Design review of the part built by this model. Coordinates are the model's own, in mm. Face numbers are marked on the shaded views. A direction names the side the tool comes from. Coordinates: 2 decimals unless noted, no trailing zeros. Write each loop counter-clockwise with the first axis right and the second up, starting at its lowest first coordinate (ties: lowest second). Pieces come first, ordered by that corner, then holes.
Solid Edge part; units mm, degrees
sketch "Sketch1" plane through (0, 0, 0) normal (0, -1, 0) x (1, 0, 0)
  line L0 (0, 12) -> (6, 12)
  line L1 (6, 12) -> (6, 10)
  line L2 (6, 10) -> (4, 10)
  line L3 (4, 10) -> (4, 0)
  line L4 (4, 0) -> (0, 0)
  line L5 (0, 0) -> (0, 12)
revolve "RevolvedProtrusion1" add sketch "Sketch1" angle 360 about axis through (0, 0, 0) along (0, 0, 1)
chamfer "Chamfer1" distance 1.5 angle 45 1 edges at (-6, 0, 12)
chamfer "Chaflán_2" distance 0.5 angle 45 1 edges at (-4, 0, 0)
sketch "Sketch2" plane through (0, 0, 10) normal (0, 0, -1) x (1, 0, 0)
  line L0 (1.5, 7) -> (-1.5, 7)
  line L1 (-1.5, 7) -> (-1.5, 5)
  line L2 (-1.5, 5) -> (1.5, 5)
  line L3 (1.5, 5) -> (1.5, 7)
extrude "VaciadoExtruido_1" cut sketch "Sketch2" against normal blind 0.5
pattern_circular "Pattern1" count 3 over 360 about axis through (0, 0, 10) along (0, 0, -1) of "VaciadoExtruido_1"
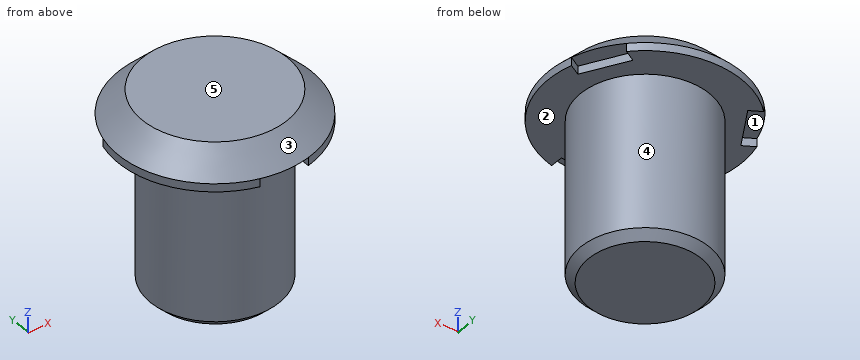
(1) Consider section B-B (y = 0). Give the boundary of the cut face in (x, z).
(2) Wall thickness on line 1 (Y direction, x = 0, z = 3.5); line 2 (Z direction, x = -0.5, y = -4); line 3 (Z direction, x = -4.25, y = -4): over which ranges is each line inside the solid? List them lowest first.
(3) For the marked faces 4 and 5, list the 3-axis set-ups (+Z, -Z, +X, -X, +Y, -Y) from which the entire face can be reached by the end or side of a thin tool; tool diameter is ignored.
(4) Mouldability with a two-part tool opening along Y and no side actions: class the marked faces 1, 2 and 3 as +Y half, -Y half, draft (parallel to the pull), parting line (faces both ways), or undercut.
(5) Consider section C-C (z = 3.25). Give the boundary of the cut face in (x, y), plus the area to 3 significant figures.
(6) Insertion check: pin 1 Ø0.8 at (x, y) = (0, -5.5) entering from -Z; pin 2 Ø3 at (x, z) = (-1, 8) entering from -Y; pin 3 Ø1.5 at (y, z) = (-3, 3.5) entering from -X. Each pin has a flat end and moves straight along its axis. Give the tip position at first contact, or say it passes through.
(7) Consider section A-A (x = 0). Give the boundary of the cut face in (y, z).
Results:
1. outline: (-6, 10) - (-4, 10) - (-4, 0.5) - (-3.5, 0) - (3.5, 0) - (4, 0.5) - (4, 10) - (6, 10) - (6, 10.5) - (4.5, 12) - (-4.5, 12) - (-6, 10.5) - close
2. line 1: y = -4 to 4
2. line 2: z = 10 to 12
2. line 3: z = 10 to 10.66
3. face 4: -Z
3. face 5: +Z, +X, -X, +Y, -Y
4. face 1: undercut
4. face 2: draft
4. face 3: parting line
5. outline: circle Ø8 at (0, 0)
5. area: 50.3 mm2
6. pin 1: stops at z = 10.5
6. pin 2: stops at y = -4
6. pin 3: stops at x = -3.31
7. outline: (-6, 10.5) - (-5, 10.5) - (-5, 10) - (-4, 10) - (-4, 0.5) - (-3.5, 0) - (3.5, 0) - (4, 0.5) - (4, 10) - (6, 10) - (6, 10.5) - (4.5, 12) - (-4.5, 12) - close
